Source: CAD feature listing. Evaluate the final solid. Frame: model axes, mm. A direction names the side the tool comes from. Give positions to 0.01 mm unless a question says otherwise; leave off trailing zeros. Loops run counter-clockwise (first coordinate to the right, second up) from the corner with the lowest first, then second, coordinate; pieces in that order, holes last.
```python
from build123d import *

# Parameters (mm, degrees)
SKETCH_1_W          = 18.5
SKETCH_1_H          = 13
EXTRUDE_1_DEPTH     = 13
SKETCH_2_R          = 4.5
CUT_EXTRUDE_1_DEPTH = 2
CUT_EXTRUDE_START   = -2
SKETCH_2_3_R        = 4.75
SKETCH_2_3_R_2      = 4.5
CUT_EXTRUDE_2_DEPTH = 14.9
SKETCH_3_W          = 3.5
SKETCH_3_H          = 9.5
CUT_EXTRUDE_3_DEPTH = 11.7
SKETCH_4_W          = 6.35
SKETCH_4_H          = 13
SKETCH_4_W_2        = 2.9
EXTRUDE_2_DEPTH     = 3
SKETCH_4_3_W        = 2.9
SKETCH_4_3_H        = 13
EXTRUDE_3_DEPTH     = 7
FILLET_1_R          = 1.5


with BuildPart() as part:
    # Sketch 1 → Extrude 1 (new body)
    with BuildSketch(Plane.XY):
        with Locations((7.25, 4.7)):
            Rectangle(SKETCH_1_W, SKETCH_1_H)
    extrude(amount=EXTRUDE_1_DEPTH)

    # Sketch 2 → Cut-Extrude 1 (cut)
    with BuildSketch(Plane(origin=(16.5, 0, 0), x_dir=(0, 0, -1), z_dir=(1, 0, 0))):
        with Locations((-6.05, 4.75)):
            Circle(SKETCH_2_R)
    extrude(amount=-CUT_EXTRUDE_1_DEPTH, mode=Mode.SUBTRACT)

    # Sketch 2_3 → Cut-Extrude 2 (cut)
    # profile 1 of 3: a face of its own
    with BuildSketch(Plane(origin=(16.5, 0, 0), x_dir=(0, 0, -1), z_dir=(1, 0, 0)).offset(CUT_EXTRUDE_START)):
        with BuildLine():
            Line((0, 9.5), (-6.05, 9.5))
            ThreePointArc((-6.05, 9.5), (-2.691242789, 8.108757211), (-1.3, 4.75))
            ThreePointArc((-1.3, 4.75), (-2.691242789, 1.391242789), (-6.05, 0))
            Line((-6.05, 0), (0, 0))
            Line((0, 0), (0, 9.5))
        make_face()
    # profile 2 of 3: a face of its own
    with BuildSketch(Plane(origin=(16.5, 0, 0), x_dir=(0, 0, -1), z_dir=(1, 0, 0)).offset(CUT_EXTRUDE_START)):
        with Locations((-6.05, 4.75)):
            Circle(SKETCH_2_3_R)
        with Locations((-6.05, 4.75)):
            Circle(SKETCH_2_3_R_2, mode=Mode.SUBTRACT)
    # profile 3 of 3: a face of its own
    with BuildSketch(Plane(origin=(16.5, 0, 0), x_dir=(0, 0, -1), z_dir=(1, 0, 0)).offset(CUT_EXTRUDE_START)):
        with Locations((-6.05, 4.75)):
            Circle(SKETCH_2_3_R_2)
    extrude(amount=-CUT_EXTRUDE_2_DEPTH, mode=Mode.SUBTRACT)

    # Sketch 3 → Cut-Extrude 3 (cut)
    with BuildSketch(Plane(origin=(0, 0, 0), x_dir=(-1, 0, 0), z_dir=(0, 0, -1))):
        with Locations((-12.75, 4.75)):
            Rectangle(SKETCH_3_W, SKETCH_3_H)
    extrude(amount=-CUT_EXTRUDE_3_DEPTH, mode=Mode.SUBTRACT)

    # Sketch 4 → Extrude 2 (add)
    with BuildSketch(Plane(origin=(0, -1.8, 0), x_dir=(1, 0, 0), z_dir=(0, 1, 0))):
        with BuildLine():
            Line((10.15, 0), (16.5, 0))
            Line((16.5, 0), (16.5, 16))
            Line((16.5, 16), (7.25, 16))
            Line((7.25, 16), (7.25, 13.3))
            ThreePointArc((7.25, 13.3), (8.876345597, 12.626345597), (9.55, 11))
            ThreePointArc((9.55, 11), (8.876345597, 9.373654403), (7.25, 8.7))
            Line((7.25, 8.7), (7.25, 0))
            Line((7.25, 0), (10.15, 0))
        make_face()
        with BuildLine():
            Line((4.35, 0), (7.25, 0))
            Line((7.25, 0), (7.25, 8.7))
            ThreePointArc((7.25, 8.7), (4.95, 11), (7.25, 13.3))
            Line((7.25, 13.3), (7.25, 16))
            Line((7.25, 16), (-2, 16))
            Line((-2, 16), (-2, 0))
            Line((-2, 0), (4.35, 0))
        make_face()
        with Locations((1.175, -6.5)):
            Rectangle(SKETCH_4_W, SKETCH_4_H)
        with Locations((13.325, -6.5)):
            Rectangle(SKETCH_4_W, SKETCH_4_H)
        with Locations((8.7, -6.5)):
            Rectangle(SKETCH_4_W_2, SKETCH_4_H)
        with Locations((5.8, -6.5)):
            Rectangle(SKETCH_4_W_2, SKETCH_4_H)
    extrude(amount=-EXTRUDE_2_DEPTH)

    # Sketch 4_3 → Extrude 3 (add)
    with BuildSketch(Plane(origin=(0, -1.8, 0), x_dir=(1, 0, 0), z_dir=(0, 1, 0))):
        with Locations((5.8, -6.5)):
            Rectangle(SKETCH_4_3_W, SKETCH_4_3_H)
        with Locations((8.7, -6.5)):
            Rectangle(SKETCH_4_3_W, SKETCH_4_3_H)
    extrude(amount=-EXTRUDE_3_DEPTH)

    # Fillet 1
    fillet_1_edges = [part.edges().sort_by_distance(p)[0] for p in [
        (10.15, -8.8, 6.5),
        (4.35, -8.8, 6.5),
        (16.5, -3.3, -16),
        (-2, -3.3, -16),
        (-2, -1.8, -8),
        (16.5, -1.8, -8),
        (16.5, 11.2, 6.5),
        (-2, 11.2, 6.5),
    ]]
    fillet(fillet_1_edges, radius=FILLET_1_R)


solid = part.part
```
(1) First-contact query: pin 1 (3 mm diameter, centred on x = 7.5, y = -7, fed in from -Z); pin 2 (3 mm diameter, centred on y = -6.5, z = -4, fed in from -X); pin 3 (1.3 mm diameter, centred on y = -6, z = 6.5, fed in from +X); pin 4 (1.8 mm diameter, centred on x = 13.5, y = 4, fed in from -Z). Flat tips, straight axial feed; report the tip coordinate or a pass-through.
A:
pin 1: stops at z = 0
pin 2: passes through
pin 3: stops at x = 10.15
pin 4: stops at z = 11.7
(2) Ray query, line 1 along Y through (x, z) = (10.5, 3.25); line 2 along X through (y, z) = (2.75, 0.5); line 3 along Y through (x, z) = (4.5, -11.25). Return the intervals inside material, ascending.
A:
line 1: y = -4.8 to 0, 9.5 to 11.2
line 2: x = -2 to -0.4, 14.5 to 16.5
line 3: y = -4.8 to -1.8
(3) Section A-A, the plane y = 4.75. Return the cut outline in (x, z).
A:
outline: (-2, 0) - (-0.4, 0) - (-0.4, 10.8) - (11, 10.8) - (11, 11.7) - (14.5, 11.7) - (14.5, 10.55) - (16.5, 10.55) - (16.5, 13) - (-2, 13) - close; (14.5, 0) - (16.5, 0) - (16.5, 1.55) - (14.5, 1.55) - close
(4) Section B-B, the plane x = 13.5. Return the cut outline in (y, z).
A:
outline: (-4.8, -16) - (-1.8, -16) - (-1.8, 0) - (0, 0) - (0, 11.7) - (9.5, 11.7) - (9.5, 0) - (11.2, 0) - (11.2, 13) - (-4.8, 13) - close
(5) Mould query, pull axis X, two halves, no side actions, for faces 6 (the flat face through (14.5, 9, 3)), 7 (the flat face through (11, 5, 11)), 8 (the cylindrical face through (-1.55, -3.65, -15.57)), 9 (the flat face through (16.5, 0, 4)). Classes: pulls with the +X half, pulls with the -X half, needs draft (parallel to the pull), parting line crosses it, or undercut.
A:
face 6: undercut
face 7: undercut
face 8: pulls with the -X half
face 9: pulls with the +X half
(6) Reachability of faces 1 (the flat face through (-0.4, 5, 5)), 2 (the cylindrical face through (-1.55, -2.23, -7.89)), 3 (the flat face through (7, -7, 0)), 4 (the flat face through (7, -1.8, -8)), 5 (the flat face through (10.15, -6, 7)) from +Z, -Z, +X, -X, +Y, -Y: full face, straight path, thin tool, end or side. Return the list, or none.
A:
face 1: -Z
face 2: -Z, -X, +Y
face 3: -Z, +X, -X, -Y
face 4: -Z, +X, -X, +Y
face 5: +Z, -Z, +X, -Y
(7) Section C-C, the plane z = -6. Return the cut outline in (x, y), then the cut area to 3 significant figures.
A:
outline: (-2, -4.8) - (16.5, -4.8) - (16.5, -3.3) arc R1.5 ccw to (15, -1.8) - (-0.5, -1.8) arc R1.5 ccw to (-2, -3.3) - close
area: 54.5 mm2
(8) Section D-D, the plane y = -4.25. Return the cut outline in (x, z).
A:
outline: (-2, -14.5) arc R1.5 ccw to (-0.5, -16) - (15, -16) arc R1.5 ccw to (16.5, -14.5) - (16.5, 13) - (-2, 13) - close; hole circle Ø4.6 at (7.25, -11)
